Geometry: final body of the model. Coordinates: model frame, mm. A direction names the side the tool comes from. Give positions to 0.01 mm unless a question says otherwise; leave off trailing zeros. Write each loop counter-clockwise with the first axis right and the second up, starting at its lowest first coordinate (ties: lowest second). Pieces come first, ordered by that corner, then holes. Notation, with made-up numbers: M 87.5,-17.5 L 146.5,-17.5 A26 cw 146.5,12.5 Z; hole C 4.5,4 d7. An arc over 180 degrees is marked long. One line per question, with ' | ' between items.
from build123d import *

# Parameters (mm, degrees)
SKETCH1_W           = 15.1
SKETCH1_H           = 3.1
BOSS_EXTRUDE1_DEPTH = 3


with BuildPart() as part:
    # Sketch1 → Boss-Extrude1 (new body)
    with BuildSketch(Plane(origin=(0, 0, 0), x_dir=(1, 0, 0), z_dir=(0, 1, 0))):
        Polygon((22.496777959, -120.1354094), (35.788574027, -113.489511367), (37.130214813, -116.17279294), (50.546622678, -109.464589007), (49.204981892, -106.781307434), (62.496777959, -100.1354094), (62.496777959, -85.8129094), (65.496777959, -85.8129094), (65.496777959, -70.8129094), (62.496777959, -70.8129094), (62.496777959, -42.1679094), (65.496777959, -42.1679094), (65.496777959, -27.1679094), (62.496777959, -27.1679094), (62.496777959, 2.411735491), (62.496777959, 26.8970906), (65.496777959, 26.8970906), (65.496777959, 41.8970906), (62.496777959, 41.8970906), (62.496777959, 70.5420906), (65.496777959, 70.5420906), (65.496777959, 85.5420906), (62.496777959, 85.5420906), (62.496777959, 99.8645906), (49.204981892, 106.510488633), (50.546622678, 109.193770206), (37.130214813, 115.901974139), (35.788574027, 113.218692566), (22.496777959, 119.8645906), (9.996777959, 119.8645906), (9.996777959, 122.8645906), (-5.003222041, 122.8645906), (-5.003222041, 119.8645906), (-30.203222041, 119.8645906), (-30.203222041, 122.8645906), (-45.203222041, 122.8645906), (-45.203222041, 119.8645906), (-57.703222041, 119.8645906), (-70.995018108, 113.218692566), (-72.336658895, 115.901974139), (-85.75306676, 109.193770206), (-84.411425973, 106.510488633), (-97.703222041, 99.8645906), (-97.703222041, 85.5420906), (-100.703222041, 85.5420906), (-100.703222041, 70.5420906), (-97.703222041, 70.5420906), (-97.703222041, 41.8970906), (-100.703222041, 41.8970906), (-100.703222041, 26.8970906), (-97.703222041, 26.8970906), (-97.703222041, 2.411735491), (-97.703222041, -27.1679094), (-100.703222041, -27.1679094), (-100.703222041, -42.1679094), (-97.703222041, -42.1679094), (-97.703222041, -70.8129094), (-100.703222041, -70.8129094), (-100.703222041, -85.8129094), (-97.703222041, -85.8129094), (-97.703222041, -100.1354094), (-84.411425973, -106.781307434), (-85.75306676, -109.464589007), (-72.336658895, -116.17279294), (-70.995018108, -113.489511367), (-57.703222041, -120.1354094), (-45.003222041, -120.1354094), (-45.003222041, -123.1354094), (-30.003222041, -123.1354094), (-30.003222041, -120.1354094), (-5.203222041, -120.1354094), (-5.203222041, -123.1354094), (9.796777959, -123.1354094), (9.796777959, -120.1354094), align=None)
        with Locations((-57.653222041, 93.700471208)):
            Rectangle(SKETCH1_W, SKETCH1_H, mode=Mode.SUBTRACT)
        with Locations((-48.060490447, -88.062310774)):
            Rectangle(SKETCH1_W, SKETCH1_H, mode=Mode.SUBTRACT)
        with Locations((22.446777959, 93.700471208)):
            Rectangle(SKETCH1_W, SKETCH1_H, mode=Mode.SUBTRACT)
        with Locations((12.854046365, -88.062310774)):
            Rectangle(SKETCH1_W, SKETCH1_H, mode=Mode.SUBTRACT)
        with BuildLine():
            Line((-67.551147117, 87.238656666), (32.344703035, 87.238656666))
            ThreePointArc((32.344703035, 87.238656666), (39.415770847, 84.309724478), (42.344703035, 77.238656666))
            Line((42.344703035, 77.238656666), (42.344703035, -71.663891856))
            ThreePointArc((42.344703035, -71.663891856), (39.415770847, -78.734959668), (32.344703035, -81.663891856))
            Line((32.344703035, -81.663891856), (-67.551147117, -81.663891856))
            ThreePointArc((-67.551147117, -81.663891856), (-74.622214928, -78.734959668), (-77.551147117, -71.663891856))
            Line((-77.551147117, -71.663891856), (-77.551147117, 77.238656666))
            ThreePointArc((-77.551147117, 77.238656666), (-74.622214928, 84.309724478), (-67.551147117, 87.238656666))
        make_face(mode=Mode.SUBTRACT)
    extrude(amount=BOSS_EXTRUDE1_DEPTH)


solid = part.part
(1) Cut plane C-C, the plane x = -9.5. Return loops of the section in (y, z).
Working result:
outline: M 0,-119.86 L 3,-119.86 L 3,-87.24 L 0,-87.24 Z; M 0,81.66 L 3,81.66 L 3,120.14 L 0,120.14 Z
(2) First-contact query: P1, Ø1.5, axis at x = -99.5, y = 1.5, coming from the +Z side; P2, Ø1.5, axis at x = -11.5, y = 2, coming from the -Z side; P3, Ø1.5, axis at y = 1, z = 94, coming from the -X side. Flat tips, straight axial feed; report the tip coordinate or a pass-through.
Working result:
P1: stops at z = 85.81 | P2: stops at z = -119.86 | P3: stops at x = -97.7
(3) Cut plane B-B, the plane x = 12.5. Return loops of the section in (y, z), then the cut area to 3 significant figures.
Working result:
outline: M 0,-119.86 L 3,-119.86 L 3,-87.24 L 0,-87.24 Z; M 0,81.66 L 3,81.66 L 3,86.51 L 0,86.51 Z; M 0,89.61 L 3,89.61 L 3,120.14 L 0,120.14 Z | area: 204 mm^2
(4) Draft query along X for faces 5 (the face through (55.944, 1.479, -103.141)), 6 (the face through (39.338, 1.479, -84.387)), 7 (the face through (-78.951, 1.479, -112.595)). Return one class per face: released by +X, released by -X, zero draft, split by the parting line, or undercut.
Working result:
face 5: released by +X | face 6: undercut | face 7: released by -X
(5) Cut plane D-D, the plane y = 1.25. Count the separate pieces of the cut face and the enclosed holes in it, then the cut area to 3 significant figures.
Working result:
separate pieces: 1 | enclosed holes: 5 | area: 17,200 mm^2
(6) Set-up query: faces 1 (the face through (-74.544, 1.479, 78.812)), 2 (the face through (29.05, 1.48, 116.86)), 3 (the face through (-64.256, 1.479, -116.588)), 4 (the face through (43.74, 1.48, 112.87)). Return all of +Z, -Z, +X, -X, +Y, -Y with unobstructed straight access to the full face (end or side cutting, diameter ignored); none if empty.
Working result:
face 1: +Y, -Y | face 2: +Z, +Y, -Y | face 3: -Z, +Y, -Y | face 4: +Z, +X, +Y, -Y
(7) Material intervals for L1, parallel to Z at x = 14.5, y = 0.8; L2, parallel to Z at x = 4, y = 0.65; L3, parallel to X at y = 2.8, z = -1, sorted ascending. Write a range as [from, to].
Working result:
L1: z = [-119.86, -87.24], [81.66, 86.51], [89.61, 120.14] | L2: z = [-122.86, -87.24], [81.66, 123.14] | L3: x = [-97.7, -77.55], [42.34, 62.5]
(8) Cut plane A-A, the plane z = 66.5. Return loops of the section in (x, y).
Working result:
outline: M -97.7,0 L -77.55,0 L -77.55,3 L -97.7,3 Z; M 42.34,0 L 62.5,0 L 62.5,3 L 42.34,3 Z
